from build123d import *

# Parameters (mm, degrees)
BOSS_EXTRUDE1_DEPTH = 16
SKETCH2_R           = 8
BOSS_EXTRUDE2_DEPTH = 29
SKETCH3_R           = 23
CUT_EXTRUDE1_DEPTH  = 16


with BuildPart() as part:
    # Sketch1 → Boss-Extrude1 (new body)
    with BuildSketch(Plane(origin=(0, 0, 0), x_dir=(0, 0, -1), z_dir=(1, 0, 0))):
        with BuildLine():
            Line((-3.203264095, 12.289389698), (91.464985163, 36.964935941))
            ThreePointArc((91.464985163, 36.964935941), (139.3, 0), (91.464985163, -36.964935941))
            Line((91.464985163, -36.964935941), (-3.203264095, -12.289389698))
            ThreePointArc((-3.203264095, -12.289389698), (-12.7, 0), (-3.203264095, 12.289389698))
        make_face()
    extrude(amount=-BOSS_EXTRUDE1_DEPTH)

    # Sketch2 → Boss-Extrude2 (add)
    with BuildSketch(Plane(origin=(0, 0, 0), x_dir=(0, 0, -1), z_dir=(1, 0, 0))):
        Circle(SKETCH2_R)
    extrude(amount=BOSS_EXTRUDE2_DEPTH)

    # Sketch3 → Cut-Extrude1 (cut)
    with BuildSketch(Plane(origin=(0, 0, 0), x_dir=(0, 0, -1), z_dir=(1, 0, 0))):
        with Locations((101.1, 0)):
            Circle(SKETCH3_R)
    extrude(amount=-CUT_EXTRUDE1_DEPTH, mode=Mode.SUBTRACT)


solid = part.part
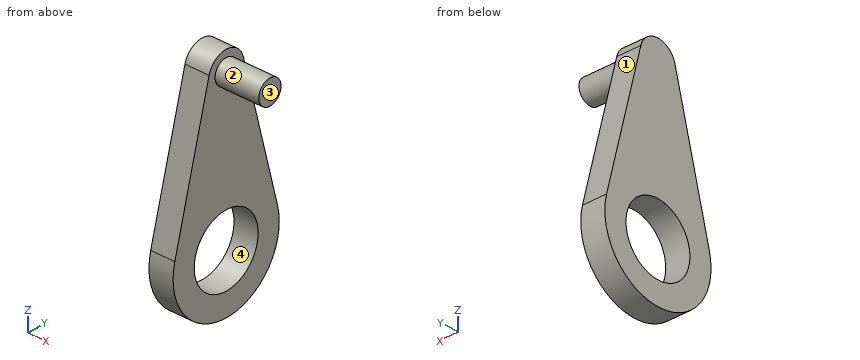
Input: part model. Units: mm. Frame: model coordinates. Face numbers are marked on the shaded views. Give positions to 0.01 mm unless a question says otherwise; leave off trailing zeros. Write each loop counter-clockwise with the first axis right and the second up, starting at its lowest first coordinate (ties: lowest second). Pieces come first, ordered by that corner, then holes. Notation, with made-up numbers: M 89.25,4 L 137.25,4 A18 ccw 137.25,22 Z; hole C 44.5,24 d11. An arc over 180 degrees is marked long. Write item = value, one per line. Start each with the question number.
1) Cut plane D-D on z = 0. Return the cut outline in (x, y).
2) Cut plane C-C on x = -12. Return the cut outline in (y, z).
3) Material intervals for line 1 along Y through (x, z) = (-5, -101.1); line 2 along X through (y, z) = (-5, -128); line 3 along Y through (x, z) = (-13, -112), sorted ascending. Write a range as [from, to].
4) Draft query along Y for the marked faces 1, 2, 3 and 4. Return one class per face: +Y half, -Y half, draft (parallel to the pull), parting line (faces both ways), or undercut.
5) Cut plane B-B on z = -101.1. Return the cut outline in (x, y), then the cut area to 3 significant figures.
6) Cut plane A-A on y = 0. Return the cut outline in (x, z).
7) First-contact query: pin 1 Ø4 at (x, z) = (-1.5, -8.5) entering from +Y; pin 2 Ø1.5 at (x, z) = (-8, -60) entering from +Y; pin 3 Ø5 at (x, y) = (-11, -4.5) entering from +Z; pin 4 Ø6 at (y, z) = (17, -91.5) entering from -X. Flat tips, straight axial feed; report the tip coordinate or a pass-through.
Solved:
q1.outline = M -16,-13.12 L 0,-13.12 L 0,-8 L 29,-8 L 29,8 L 0,8 L 0,13.12 L -16,13.12 Z
q2.outline = M -36.96,-91.46 A38.2 ccw long 36.96,-91.46 L 12.29,3.2 A12.7 ccw -12.29,3.2 Z; hole C 0,-101.1 d46
q3.line_1 = [-38.2, -23], [23, 38.2]
q3.line_2 = [-16, 0]
q3.line_3 = [-36.61, -20.25], [20.25, 36.61]
q4.face_1 = +Y half
q4.face_2 = parting line
q4.face_3 = draft
q4.face_4 = undercut
q5.outline = M -16,-38.2 L 0,-38.2 L 0,-23 L -16,-23 Z; M -16,23 L 0,23 L 0,38.2 L -16,38.2 Z
q5.area = 486 mm2
q6.outline = M -16,-139.3 L 0,-139.3 L 0,-124.1 L -16,-124.1 Z; M -16,-78.1 L 0,-78.1 L 0,-8 L 29,-8 L 29,8 L 0,8 L 0,12.7 L -16,12.7 Z
q7.pin_1 = 15.86
q7.pin_2 = 28.96
q7.pin_3 = 12.54
q7.pin_4 = through
